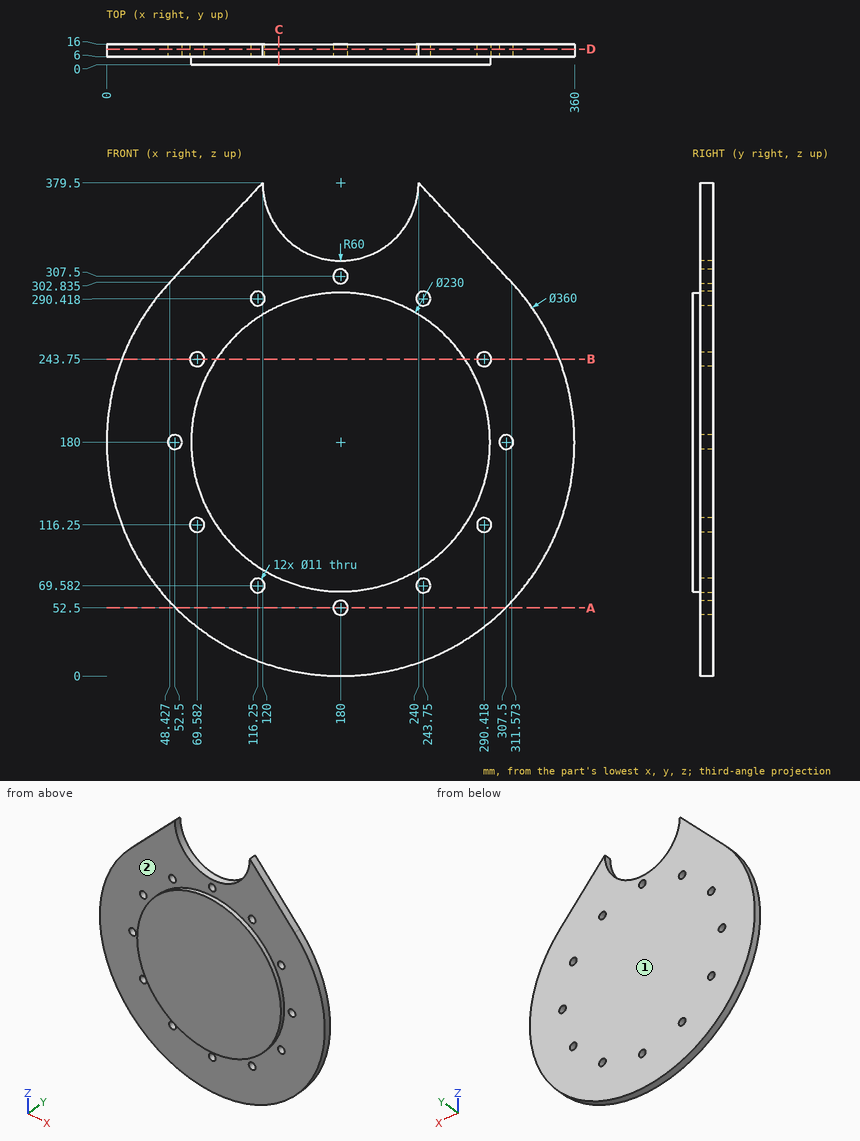
Design review of the part shown in the three views and the two pictorial views. Dimensions are in mm from the part's minimum x, y and z. A direction names the side the tool comes from. Give positions to 0.01 mm unless a question says otherwise; leave off trailing zeros. Order: outer loops, then holes, each group sorted by start corner. A loop starts at its lowest first (then second) coordinate and runs counter-clockwise, first axis right, second up. Notation, with made-up numbers: (44, 28) -> (93, 28) arc R18 cw to (93, 35) -> close; hole circle Ø1 at (12.5, 72.25). An arc over 180 degrees is marked (long way). Write each question's results on one line, items separated by ' | '. Start each with the question number.
Q1. Add section A-A on z = 52.5. Give the boundary of the cut face in (x, y).
Q2. Add section C-C on x = 132.5. Give the boundary of the cut face in (y, z), and give its area (3 significant figures).
Q3. For pin 1 (2 mm diameter, centred on y = 14, z = 83.5, fed in from +X); pin 2 (6 mm diameter, centred on y = 12.5, z = 133, fed in from -X); pin 3 (3 mm diameter, centred on x = 299, z = 126, fed in from -Y), all flat-tipped, find the tip position at first contact; note any pin that passes through.
Q4. Wall thickness on L1, parallel to Y at x = 293, z = 237; L2, parallel to Z at x = 248, y = 10 (1 decimal); L3, parallel to Z at x = 307.5, y = 9.75: over which ranges is each line inside the solid? List them lowest first. Write a range as from..to.
Q5. Add section B-B on z = 243.75. Give the boundary of the cut face in (x, y).
Q6. Machinability: for the marked faces 1 and 2, which of the approach directions +Z, -Z, +X, -X, +Y, -Y give a long, thin tool a straight path to every point of the face, cutting with its end or side? Answer none if there is none.
Q7. Add section D-D on y = 12. State how many separate pieces and enclosed holes the cut face has, and give its area (3 significant figures).
Found:
1) outline: (52.94, 6) -> (174.5, 6) -> (174.5, 16) -> (52.94, 16) -> close; (185.5, 6) -> (307.06, 6) -> (307.06, 16) -> (185.5, 16) -> close
2) outline: (0, 75.27) -> (6, 75.27) -> (6, 6.38) -> (16, 6.38) -> (16, 342.84) -> (6, 342.84) -> (6, 284.73) -> (0, 284.73) -> close | area: 4,620 mm2
3) pin 1: stops at x = 332.58 | pin 2: stops at x = 5.46 | pin 3: stops at y = 6
4) L1: y = 6..16 | L2: z = 13.3..66.1, 73.1..286.9, 293.9..370.9 | L3: z = 52.94..174.5, 185.5..307.2
5) outline: (11.67, 6) -> (64.08, 6) -> (64.08, 16) -> (11.67, 16) -> close; (75.08, 6) -> (84.29, 6) -> (84.29, 0) -> (275.71, 0) -> (275.71, 6) -> (284.92, 6) -> (284.92, 16) -> (75.08, 16) -> close; (295.92, 6) -> (348.33, 6) -> (348.33, 16) -> (295.92, 16) -> close
6) face 1: +Z, -Z, +X, -X, +Y | face 2: -Y
7) separate pieces: 1 | enclosed holes: 12 | area: 99,300 mm2
